Work out the finished part from the listing and answer in its coordinate system (mm). Give positions to 0.01 mm unless a question says otherwise; leave off trailing zeros. Loops run counter-clockwise (first coordinate to the right, second up) from the corner with the lowest first, then second, coordinate; pieces in that order, holes last.
```python
from build123d import *

# Parameters (mm, degrees)
F1_R            = 25
F1_R_2          = 3.25
F2_DEPTH        = 2
F1_R_3          = 30
F3_DEPTH        = 1
F4_DEPTH        = 25
F4_COPIES_COUNT = 3


# Not quite as in the source:
# - a pattern or mirror of a feature is missing from the dataset's text; its kind, count and spacing are read off the source's solid


with BuildPart() as f2:
    # F1 (on Top) → F2 (new body)
    with BuildSketch(Plane.XY):
        Circle(F1_R)
        with Locations((0, 12.5)):
            Circle(F1_R_2, mode=Mode.SUBTRACT)
        with Locations((0, 12.5)):
            Circle(F1_R_2)
    extrude(amount=-F2_DEPTH)

    # F1 (on Top) → F3 (join)
    with BuildSketch(Plane.XY):
        Circle(F1_R_3)
        Circle(F1_R, mode=Mode.SUBTRACT)
    extrude(amount=-F3_DEPTH)

    # F1 (on Top) → F4 (cut)
    with BuildSketch(Plane.XY):
        with Locations((0, 12.5)):
            Circle(F1_R_2)
    f4 = extrude(amount=-F4_DEPTH, mode=Mode.SUBTRACT)

    # F4_copies: F4 ×3 about axis
    f4_copies_axis = Axis((0, 0, 0), (0, 0, 1))
    for i in range(1, F4_COPIES_COUNT):
        add(f4.rotate(f4_copies_axis, i * 360 / F4_COPIES_COUNT), mode=Mode.SUBTRACT)


solid = f2.part
```
Q1. Section D-D on y = 0 is taken. Give the vertices of the cut face in (x, z), plus the area to 3 significant figures.
Q2. Section C-C on y = -6.25 is taken. Give the vertices of the cut face in (x, z), plus the area to 3 significant figures.
Q3. Section B-B on y = 11.5 is taken. Give the vertices of the cut face in (x, z).
Q4. Consider line 1 along Y through (x, z) = (0, -1.5); line 2 along X through (y, z) = (-6.5, -0.45); line 3 along X through (y, z) = (-8, -0.9). Determine where each line is inside the solid, lowest interval first.
Q5. Given pin 1 (4 mm diameter, centred on x = 0, y = 12.5, fed in from +Z), flat-ended and moving along its own axis, determine where the tip first touches the part or whether it passes through.
Q6. Determine the mould class of faces 1 (the face through (-7.82, -7.49, -0.99)), 2 (the face through (-7, 25, -1)), 3 (the face through (23.846, 7.509, -1.493)), 4 (the face through (-0.423, 15.722, -0.986)) for opening direction X: +X half, -X half, draft (parallel to the pull), parting line (faces both ways), or undercut.
Q7. Section A-A on x = 0 is taken. Give the vertices of the cut face in (y, z), plus the area to 3 significant figures.
Check result:
1. outline: (-30, -1) - (-25, -1) - (-25, -2) - (25, -2) - (25, -1) - (30, -1) - (30, 0) - (-30, 0) - close
1. area: 110 mm2
2. outline: (-29.34, -1) - (-24.21, -1) - (-24.21, -2) - (-14.08, -2) - (-14.08, 0) - (-29.34, 0) - close; (-7.58, -2) - (7.58, -2) - (7.58, 0) - (-7.58, 0) - close; (14.08, -2) - (24.21, -2) - (24.21, -1) - (29.34, -1) - (29.34, 0) - (14.08, 0) - close
2. area: 81.1 mm2
3. outline: (-27.71, -1) - (-22.2, -1) - (-22.2, -2) - (-3.09, -2) - (-3.09, 0) - (-27.71, 0) - close; (3.09, -2) - (22.2, -2) - (22.2, -1) - (27.71, -1) - (27.71, 0) - (3.09, 0) - close
4. line 1: y = -25 to 9.25, 15.75 to 25
4. line 2: x = -29.29 to -14.07, -7.58 to 7.58, 14.07 to 29.29
4. line 3: x = -28.91 to -13.56, -8.09 to 8.09, 13.56 to 28.91
5. pin 1: passes through
6. face 1: undercut
6. face 2: draft
6. face 3: parting line
6. face 4: undercut
7. outline: (-30, -1) - (-25, -1) - (-25, -2) - (9.25, -2) - (9.25, 0) - (-30, 0) - close; (15.75, -2) - (25, -2) - (25, -1) - (30, -1) - (30, 0) - (15.75, 0) - close
7. area: 97.0 mm2
